```python
from build123d import *

# Parameters (mm, degrees)
F0_R     = 3.175
F0_R_2   = 1.5875
F1_DEPTH = 3.048


with BuildPart() as f1:
    # F0 (on Front) → F1 (new body)
    with BuildSketch(Plane.XZ):
        with BuildLine():
            ThreePointArc((-9.525, 0), (0, 9.525), (9.525, 0))
            Line((9.525, 0), (36.5125, 0))
            ThreePointArc((36.5125, 0), (38.605385, 5.370697), (43.780377, 7.909204))
            Line((43.780377, 7.909204), (19.011896, 7.909204))
            ThreePointArc((19.011896, 7.909204), (13.137807, 10.502095), (11.095287, 16.589469))
            Line((11.095287, 16.589469), (15.754219, 61.545461))
            ThreePointArc((15.754219, 61.545461), (-0.178582, 47.626004), (-15.794203, 61.90038))
            Line((-15.794203, 61.90038), (-9.525, 0))
        make_face()
        with BuildLine():
            ThreePointArc((0.677344, -9.500886), (6.970557, -6.491299), (9.525, 0))
            ThreePointArc((9.525, 0), (0, 9.525), (-9.525, 0))
            ThreePointArc((-9.525, 0), (-6.735192, -6.735192), (0, -9.525))
            Line((0, -9.525), (0.677344, -9.500886))
        make_face()
        with BuildLine():
            Line((36.5125, 0), (9.525, 0))
            ThreePointArc((9.525, 0), (6.970557, -6.491299), (0.677344, -9.500886))
            Line((0.677344, -9.500886), (44.732405, -7.932475))
            ThreePointArc((44.732405, -7.932475), (38.93809, -5.711633), (36.5125, 0))
        make_face()
        with BuildLine():
            ThreePointArc((47.625, 0), (44.45, 3.175), (41.275, 0))
            ThreePointArc((41.275, 0), (44.45, -3.175), (47.625, 0))
        make_face()
        with BuildLine():
            ThreePointArc((43.780377, 7.909204), (38.605385, 5.370697), (36.5125, 0))
            ThreePointArc((36.5125, 0), (38.93809, -5.711633), (44.732405, -7.932475))
            ThreePointArc((44.732405, -7.932475), (50.161633, -5.51191), (52.3875, 0))
            ThreePointArc((52.3875, 0), (49.820697, 5.844615), (43.780377, 7.909204))
        make_face()
        with BuildLine():
            ThreePointArc((47.625, 0), (44.45, -3.175), (41.275, 0))
            ThreePointArc((41.275, 0), (44.45, 3.175), (47.625, 0))
        make_face(mode=Mode.SUBTRACT)
        with BuildLine():
            ThreePointArc((0, -9.525), (0.338886, -9.51897), (0.677344, -9.500886))
            Line((0.677344, -9.500886), (0, -9.525))
        make_face()
        with BuildLine():
            ThreePointArc((-15.654504, 66.13669), (-15.866375, 64.023219), (-15.794203, 61.90038))
            ThreePointArc((-15.794203, 61.90038), (-0.178582, 47.626004), (15.754219, 61.545461))
            ThreePointArc((15.754219, 61.545461), (15.844776, 62.520866), (15.875, 63.5))
            ThreePointArc((15.875, 63.5), (15.821396, 64.803473), (15.660948, 66.098142))
            ThreePointArc((15.660948, 66.098142), (0.019541, 79.374988), (-15.654504, 66.13669))
        make_face()
        with Locations((0, 63.5)):
            Circle(F0_R, mode=Mode.SUBTRACT)
        with BuildLine():
            Line((-9.402802, 103.254165), (-15.654504, 66.13669))
            ThreePointArc((-15.654504, 66.13669), (0.019541, 79.374988), (15.660948, 66.098142))
            Line((15.660948, 66.098142), (9.44669, 103.556119))
            ThreePointArc((9.44669, 103.556119), (0.152563, 95.251222), (-9.402802, 103.254165))
        make_face()
        with Locations((-1.5875, 91.382228)):
            Circle(F0_R_2, mode=Mode.SUBTRACT)
        with BuildLine():
            Line((-8.385852, 109.29198), (-9.402802, 103.254165))
            ThreePointArc((-9.402802, 103.254165), (0.152563, 95.251222), (9.44669, 103.556119))
            Line((9.44669, 103.556119), (8.547032, 108.979029))
            ThreePointArc((8.547032, 108.979029), (0.176009, 114.298374), (-8.385852, 109.29198))
        make_face()
        with Locations((0, 104.775)):
            Circle(F0_R, mode=Mode.SUBTRACT)
        with BuildLine():
            ThreePointArc((-8.385852, 109.29198), (-9.392702, 106.357014), (-9.402802, 103.254165))
            Line((-9.402802, 103.254165), (-8.385852, 109.29198))
        make_face()
        with BuildLine():
            Line((8.547032, 108.979029), (9.44669, 103.556119))
            ThreePointArc((9.44669, 103.556119), (9.505402, 104.164303), (9.525, 104.775))
            ThreePointArc((9.525, 104.775), (9.277287, 106.933141), (8.547032, 108.979029))
        make_face()
    extrude(amount=F1_DEPTH)


solid = f1.part
```
CAD build for the part. Positions are in the model's coordinates, mm. A direction names the side the tool comes from. Coordinates: 2 decimals unless noted, no trailing zeros. Write each loop counter-clockwise with the first axis right and the second up, starting at its lowest first coordinate (ties: lowest second). Pieces come first, ordered by that corner, then holes. Notation, with made-up numbers: (-11, 21.5) -> (42, 21.5) arc R29 ccw to (42, 48.5) -> close; hole circle Ø3 at (67, -5.5). An arc over 180 degrees is marked (long way). Return JSON: item names as keys, results as strings. Group by question number.
Q1. Cut at B-B, the plane x = 22.5. Give the cut face in (y, z), then the cut area to 3 significant figures.
Q2. Flat gauge pins, fed straight in: pin 1 (4 mm diameter, centred on x = 0, z = 63.5, fed in from +Y); pin 2 (1 mm diameter, centred on x = 39.5, y = -2, fed in from +Z); pin 3 (1.5 mm diameter, centred on y = -0.5, z = 79.5, fed in from -X). Where does each tip first touch, or does it go through?
Q3. Cut at C-C, the plane z = 55. Give the cut face in (x, y), then the cut area to 3 significant figures.
Q4. Drill centre lines: line 1 (Z direction, x = 45, y = -1.85); line 2 (Z direction, x = 44.45, y = -1.35) (1 decimal); line 3 (X direction, y = -1.65, z = 1.5). Where is each one in solid material? Low to high.
Q5. Cut at A-A, the plane y = -0.65. State how many separate pieces and enclosed holes the cut face has, then the cut area to 3 significant figures.
Q6. Which spindle directions (+Z, -Z, +X, -X, +Y, -Y) get a long thin tool onto all of the face, cutting with end or side? Do faces 1 (the face through (3, 0, 39)), 2 (the face through (13.39, -1.5, 38.75)). Say none if no direction does.
Q7. Pull direction Z, two halves, no side cores. Call faces 3 (the face through (-15.865, -1.503, 64.053)), 4 (the face through (3, -3.048, 39)), 5 (the face through (-0.688, -1.503, 101.676)): released by +Z, released by -Z, zero draft, split by the parting line, or undercut.
Returned:
{
 "1": {"outline": "(-3.05, -8.72) -> (0, -8.72) -> (0, 7.91) -> (-3.05, 7.91) -> close", "area": "50.7 mm2"},
 "2": {"pin 1": "passes through", "pin 2": "stops at z = 7.91", "pin 3": "stops at x = -13.53"},
 "3": {"outline": "(-15.1, -3.05) -> (15.08, -3.05) -> (15.08, 0) -> (-15.1, 0) -> close", "area": "92.0 mm2"},
 "4": {"line 1": "z = -7.92 to -3.13, 3.13 to 7.92", "line 2": "z = -7.9 to -3.2, 3.2 to 7.9", "line 3": "x = -9.68 to 41.65, 47.25 to 52.24"},
 "5": {"separate pieces": "1", "enclosed holes": "4", "area": "3,550 mm2"},
 "6": {"face 1": "+Z, -Z, +X, -X, +Y", "face 2": "+X, +Y, -Y"},
 "7": {"face 3": "split by the parting line", "face 4": "zero draft", "face 5": "undercut"}
}
